Here's the drawing with two shaded views (mm, measured from the low corner). I have some questions. Coordinates: 2 decimals unless noted, no trailing zeros. Write each loop counter-clockwise with the first axis right and the second up, starting at its lowest first coordinate (ties: lowest second). Pieces come first, ordered by that corner, then holes. Notation, with made-up numbers: M 51,47 L 63,47 A27 ccw 63,69 Z; hole C 59.5,27 d7. An arc over 180 degrees is marked long. Use one line per item in the form item = value. Start each with the question number.
1. Thinking about a two-plate mould opening in X: for the marked faces 1 and 2, which applies, released by +X, released by -X, zero draft, split by the parting line, or undercut?
2. Please list where these lines run through material, in increasing order: line 1 along Y through (x, z) = (13, 7); line 2 along Z through (x, y) = (10.25, 14.25); line 3 along Z through (x, y) = (5.25, 5.75). Write a range as [from, to].
3. I want a section at A-A, the plane x = 6.85. List the corners of the cut face in (y, z) for me, plus the area to 3 significant figures.
4. I'm going to push flat-ended pins straight in: pin 1 Ø3 at (x, y) = (3.5, 15) entering from -Z; pin 2 Ø2 at (y, z) = (3, 3.5) entering from -X; pin 3 Ø3 at (y, z) = (12, 7.5) entering from +X. Where does each tip first touch, or does it pass through?
5. I want a section at B-B, the plane z = 6.85. List the corners of the cut face in (x, y) for me, plus the area to 3 significant figures.
6. I want a section at D-D, the plane y = 8.5. List the corners of the cut face in (x, z) for me, plus the area to 3 significant figures.
7. I want a section at C-C, the plane y = 16.25. List the corners of the cut face in (x, z) for me.
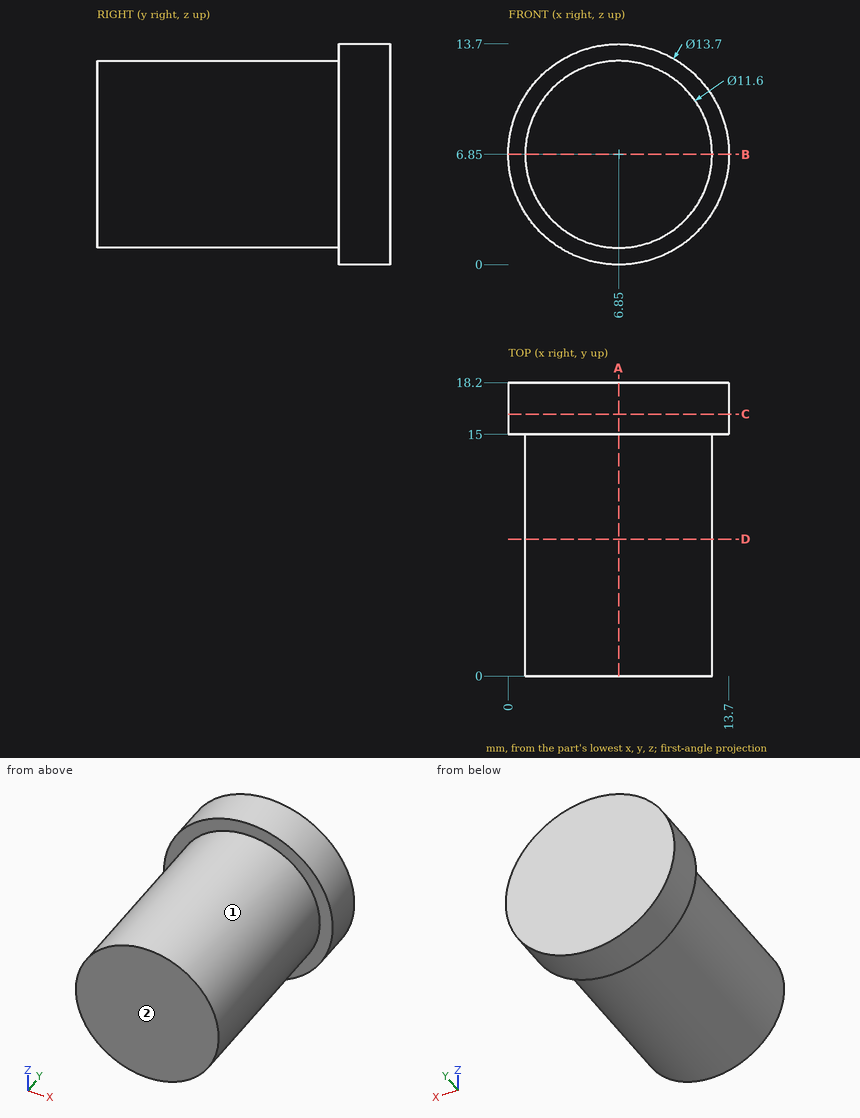
Answer list:
q1.face_1 = split by the parting line
q1.face_2 = zero draft
q2.line_1 = [15, 18.2]
q2.line_2 = [2.15, 11.55]
q2.line_3 = [1.28, 12.42]
q3.outline = M 0,1.05 L 15,1.05 L 15,0 L 18.2,0 L 18.2,13.7 L 15,13.7 L 15,12.65 L 0,12.65 Z
q3.area = 218 mm²
q4.pin_1 = 0.25
q4.pin_2 = 1.55
q4.pin_3 = 12.65
q5.outline = M 0,15 L 1.05,15 L 1.05,0 L 12.65,0 L 12.65,15 L 13.7,15 L 13.7,18.2 L 0,18.2 Z
q5.area = 218 mm²
q6.outline = C 6.85,6.85 d11.6
q6.area = 106 mm²
q7.outline = C 6.85,6.85 d13.7
